from build123d import *

# Parameters (mm, degrees)
CROQUIS1_W                         = 60
CROQUIS1_H                         = 70
BRIDA_BASE1_DEPTH                  = 1.5
BRIDA_DE_ARISTA1_STRIP_W           = 7.4732
BRIDA_DE_ARISTA1_STRIP_H           = 1.5
BRIDA_DE_ARISTA1_STRIP_CUT_DEPTH   = 70
BRIDA_DE_ARISTA1_STRIP_2_W         = 7.4732
BRIDA_DE_ARISTA1_STRIP_2_H         = 1.5
BRIDA_DE_ARISTA1_STRIP_CUT_2_DEPTH = 70
BRIDA_DE_ARISTA1_DEPTH             = 70
BRIDA_DE_ARISTA1_BEND_DEPTH        = 70
ROMPER_START                       = -40.658639918
ROMPER_ESQUINA1_OUTLINE_W          = 64
ROMPER_ESQUINA1_OUTLINE_H          = 51.123106012
ROMPER_ESQUINA1_DEPTH              = 3.535533906
ROMPER_START_2                     = 5.303300859
ROMPER_ESQUINA1_2_OUTLINE_W        = 64
ROMPER_ESQUINA1_2_OUTLINE_H        = 3.876893988
ROMPER_ESQUINA1_2_DEPTH            = 7.071067812
CROQUIS16_R                        = 2.5
CORTAR_EXTRUIR1_DEPTH              = 74.015409333


# Read off the part's stored shape, not the designer's step: Romper esquina1
# Sheet-metal steps are written as plain solids
with BuildPart() as part:
    # Croquis1 → Brida base1 (new body)
    with BuildSketch(Plane.XY):
        Rectangle(CROQUIS1_W, CROQUIS1_H)
    extrude(amount=-BRIDA_BASE1_DEPTH)

    # Brida de arista1 strip (across the edge) → Brida de arista1 strip cut (cut)
    with BuildSketch(Plane(origin=(-30, 35, 0), x_dir=(1, 0, 0), z_dir=(0, -1, 0))):
        with Locations((-1.5, -0.75)):
            Rectangle(BRIDA_DE_ARISTA1_STRIP_W, BRIDA_DE_ARISTA1_STRIP_H)
    extrude(amount=BRIDA_DE_ARISTA1_STRIP_CUT_DEPTH, mode=Mode.SUBTRACT)

    # Brida de arista1 strip 2 (across the edge) → Brida de arista1 strip cut 2 (cut)
    with BuildSketch(Plane(origin=(30, -35, 0), x_dir=(-1, 0, 0), z_dir=(0, 1, 0))):
        with Locations((-1.5, -0.75)):
            Rectangle(BRIDA_DE_ARISTA1_STRIP_2_W, BRIDA_DE_ARISTA1_STRIP_2_H)
    extrude(amount=BRIDA_DE_ARISTA1_STRIP_CUT_2_DEPTH, mode=Mode.SUBTRACT)

    # Brida de arista1 section (across the edge) → Brida de arista1 (add)
    with BuildSketch(Plane(origin=(-30, 35, 0), x_dir=(1, 0, 0), z_dir=(0, -1, 0))):
        with BuildLine():
            Line((0, 0.7366), (0, 22.5))
            Line((0, 22.5), (1.5, 22.5))
            Line((1.5, 22.5), (1.5, 0.7366))
            ThreePointArc((1.5, 0.7366), (1.715745145, 0.215745145), (2.2366, 0))
            Line((2.2366, 0), (2.2366, -1.5))
            ThreePointArc((2.2366, -1.5), (0.655084973, -0.844915027), (0, 0.7366))
        make_face()
    extrude(amount=BRIDA_DE_ARISTA1_DEPTH)

    # Brida de arista1 section 2 (across the edge) → Brida de arista1 bend (add)
    with BuildSketch(Plane(origin=(30, -35, 0), x_dir=(-1, 0, 0), z_dir=(0, 1, 0))):
        with BuildLine():
            Line((0, 0.7366), (0, 22.5))
            Line((0, 22.5), (1.5, 22.5))
            Line((1.5, 22.5), (1.5, 0.7366))
            ThreePointArc((1.5, 0.7366), (1.715745145, 0.215745145), (2.2366, 0))
            Line((2.2366, 0), (2.2366, -1.5))
            ThreePointArc((2.2366, -1.5), (0.655084973, -0.844915027), (0, 0.7366))
        make_face()
    extrude(amount=BRIDA_DE_ARISTA1_BEND_DEPTH)

    # Romper esquina1 outline → Romper esquina1 (cut)
    with BuildSketch(Plane(origin=(0, 0, 0), x_dir=(1, 0, 0), z_dir=(0, 0.707106781186548, -0.707106781186547)).offset(ROMPER_START)):
        with Locations((0, -11.561553006)):
            Rectangle(ROMPER_ESQUINA1_OUTLINE_W, ROMPER_ESQUINA1_OUTLINE_H)
    extrude(amount=ROMPER_ESQUINA1_DEPTH, mode=Mode.SUBTRACT)

    # Romper esquina1 2 outline → Romper esquina1 2 (cut)
    with BuildSketch(Plane(origin=(0, 0, 0), x_dir=(1, 0, 0), z_dir=(0, 0.707106781186548, -0.707106781186547)).offset(ROMPER_START_2)):
        with Locations((0, -39.061553006)):
            Rectangle(ROMPER_ESQUINA1_2_OUTLINE_W, ROMPER_ESQUINA1_2_OUTLINE_H)
    extrude(amount=ROMPER_ESQUINA1_2_DEPTH, mode=Mode.SUBTRACT)

    # Croquis16 → Cortar-Extruir1 (cut, through all)
    with BuildSketch(Plane(origin=(30, 0, 0), x_dir=(0, 0, -1), z_dir=(1, 0, 0))):
        with Locations((-12.5, -20)):
            Circle(CROQUIS16_R)
        with Locations((-12.5, 20)):
            Circle(CROQUIS16_R)
    extrude(amount=-CORTAR_EXTRUIR1_DEPTH, mode=Mode.SUBTRACT)


solid = part.part
Input: part model. Units: mm. Frame: model coordinates. A direction names the side the tool comes from. Give positions to 0.01 mm unless a question says otherwise; leave off trailing zeros. Write each loop counter-clockwise with the first axis right and the second up, starting at its lowest first coordinate (ties: lowest second). Pieces come first, ordered by that corner, then holes.
Q1. Section B-B, the plane y = -20. Output: boundary loops of the cut face in (x, z), plus the area to 3 significant figures.
Q2. Section C-C, the plane z = 12.5. Output: boundary loops of the cut face in (x, y).
Q3. Section A-A, the plane z = 18.5. Output: boundary loops of the cut face in (x, y).
Q4. Section D-D, the plane z = 8. Output: boundary loops of the cut face in (x, y), plus the area to 3 significant figures.
Q5. Material intervals for probe 1 along Y at (x, z) = (-28.95, 12.5); probe 2 along X at (y, z) = (3, 7); probe 3 along Z at (x, y) = (10, 23.5), sorted ascending.
Q6. Pull-direction query (Y, two-part tool) for faces 3 (the face through (28.5, 0, 12)), 4 (the face through (-0.1, 35, -0.4)), 5 (the face through (-29.24, 22.48, 12.83)); classes: pulls with the +Y half, pulls with the -Y half, needs draft (parallel to the pull), parting line crosses it, or undercut.
Q7. First-contact query: P1, Ø8, axis at y = -20, z = 12.5, coming from the -X side; P2, Ø2, axis at x = 12.5, y = 5, coming from the +Z side; P3, Ø12, axis at x = -21, z = 9.5, coming from the -Y side. Flat tips, straight axial feed; report the tip coordinate or a pass-through.
Q8. Set-up query: faces 1 (the face through (-29.3, 32.5, 20)), 2 (the face through (0, 0, 0)). Return all of +Z, -Z, +X, -X, +Y, -Y with unobstructed straight access to the full face (end or side cutting, diameter ignored); none if empty.
Filled in:
1. outline: (-30, 0.74) arc R2.24 ccw to (-27.76, -1.5) - (27.76, -1.5) arc R2.24 ccw to (30, 0.74) - (30, 10) - (28.5, 10) - (28.5, 0.74) arc R0.74 cw to (27.76, 0) - (-27.76, 0) arc R0.74 cw to (-28.5, 0.74) - (-28.5, 10) - (-30, 10) - close; (-30, 15) - (-28.5, 15) - (-28.5, 22.5) - (-30, 22.5) - close; (28.5, 15) - (30, 15) - (30, 22.5) - (28.5, 22.5) - close
1. area: 141 mm2
2. outline: (-30, -35) - (-28.5, -35) - (-28.5, -22.5) - (-30, -22.5) - close; (-30, -17.5) - (-28.5, -17.5) - (-28.5, 17.5) - (-30, 17.5) - close; (-30, 22.5) - (-28.5, 22.5) - (-28.5, 35) - (-30, 35) - close; (28.5, -35) - (30, -35) - (30, -22.5) - (28.5, -22.5) - close; (28.5, -17.5) - (30, -17.5) - (30, 17.5) - (28.5, 17.5) - close; (28.5, 22.5) - (30, 22.5) - (30, 35) - (28.5, 35) - close
3. outline: (-30, -34) - (-28.5, -34) - (-28.5, 34) - (-30, 34) - close; (28.5, -34) - (30, -34) - (30, 34) - (28.5, 34) - close
4. outline: (-30, -35) - (-28.5, -35) - (-28.5, 35) - (-30, 35) - close; (28.5, -35) - (30, -35) - (30, 35) - (28.5, 35) - close
4. area: 210 mm2
5. probe 1: y = -35 to -22.5, -17.5 to 17.5, 22.5 to 35
5. probe 2: x = -30 to -28.5, 28.5 to 30
5. probe 3: z = -1.5 to 0
6. face 3: needs draft
6. face 4: pulls with the +Y half
6. face 5: undercut
7. P1: stops at x = -30
7. P2: stops at z = 0
7. P3: passes through
8. face 1: +Z, +X, -X, +Y
8. face 2: +Z, +Y, -Y
